Geometry check sheet. Reference: the model listing, model coordinates, mm. A direction names the side the tool comes from. Give positions to 0.01 mm unless a question says otherwise; leave off trailing zeros. Loops run counter-clockwise (first coordinate to the right, second up) from the corner with the lowest first, then second, coordinate; pieces in that order, holes last. Notation, with made-up numbers: (53, 19.5) -> (85, 19.5) arc R22 ccw to (85, 57.5) -> close; hole circle Ø9 at (41.25, -29). An arc over 180 degrees is marked (long way). Answer in a Markdown table with one row per item. Add a question column.
```python
from build123d import *

# Parameters (mm, degrees)
MAIN_BODY_DEPTH     = 7
SKETCH3_W           = 32
SKETCH3_H           = 20
BOSS_EXTRUDE2_DEPTH = 7
SKETCH4_W           = 28.5
SKETCH4_H           = 4
BOSS_EXTRUDE3_DEPTH = 6.5
SKETCH7_W           = 32
SKETCH7_H           = 7
BOSS_EXTRUDE4_DEPTH = 15
SKETCH10_R          = 1.9
CUT_EXTRUDE5_DEPTH  = 7
SKETCH13_W          = 10
SKETCH13_H          = 20
BOSS_EXTRUDE5_DEPTH = 10
SKETCH14_W          = 40
SKETCH14_H          = 20
SKETCH14_R          = 1.9
BOSS_EXTRUDE6_DEPTH = 6
SKETCH17_W          = 71
SKETCH17_H          = 5
BOSS_EXTRUDE7_DEPTH = 7
SKETCH19_R          = 1.25
CUT_EXTRUDE7_DEPTH  = 7
SKETCH21_R          = 1.6
CUT_EXTRUDE9_DEPTH  = 4
SKETCH22_R          = 1.9
CUT_EXTRUDE10_DEPTH = 7
SKETCH15_R          = 2.5621
DUE_MOUNT_DEPTH     = 172.689399789


with BuildPart() as part:
    # Sketch2 → Main body (new body)
    with BuildSketch(Plane(origin=(0, 0, 0), x_dir=(1, 0, 0), z_dir=(0, 1, 0))):
        with BuildLine():
            Line((0, 0), (71, 0))
            Line((71, 0), (71, -120))
            ThreePointArc((71, -120), (35.5, -155.5), (0, -120))
            Line((0, -120), (0, 0))
        make_face()
    extrude(amount=MAIN_BODY_DEPTH)

    # Sketch3 → Boss-Extrude2 (add)
    with BuildSketch(Plane(origin=(0, 7, 0), x_dir=(1, 0, 0), z_dir=(0, 1, 0))):
        with Locations((35.5, 10)):
            Rectangle(SKETCH3_W, SKETCH3_H)
    extrude(amount=-BOSS_EXTRUDE2_DEPTH)

    # Sketch4 → Boss-Extrude3 (add)
    with BuildSketch(Plane(origin=(0, 7, 0), x_dir=(1, 0, 0), z_dir=(0, 1, 0))):
        with Locations((35.5, 18)):
            Rectangle(SKETCH4_W, SKETCH4_H)
    extrude(amount=BOSS_EXTRUDE3_DEPTH)

    # Sketch7 → Boss-Extrude4 (add)
    with BuildSketch(Plane(origin=(0, 0, -20), x_dir=(-1, 0, 0), z_dir=(0, 0, -1))):
        with Locations((-35.5, 3.5)):
            Rectangle(SKETCH7_W, SKETCH7_H)
    extrude(amount=BOSS_EXTRUDE4_DEPTH)

    # Sketch10 → Cut-Extrude5 (cut)
    with BuildSketch(Plane(origin=(0, 7, 0), x_dir=(1, 0, 0), z_dir=(0, 1, 0))):
        with Locations(Location((4, -120, 0), (0, 0, 270))):
            Circle(SKETCH10_R)
        with Locations(Location((4, -110, 0), (0, 0, 270))):
            Circle(SKETCH10_R)
        with Locations(Location((4, -100, 0), (0, 0, 270))):
            Circle(SKETCH10_R)
        with Locations(Location((4, -90, 0), (0, 0, 270))):
            Circle(SKETCH10_R)
        with Locations(Location((4, -80, 0), (0, 0, 270))):
            Circle(SKETCH10_R)
        with Locations(Location((4, -70, 0), (0, 0, 270))):
            Circle(SKETCH10_R)
        with Locations(Location((4, -60, 0), (0, 0, 270))):
            Circle(SKETCH10_R)
        with Locations(Location((4, -50, 0), (0, 0, 270))):
            Circle(SKETCH10_R)
        with Locations(Location((4, -40, 0), (0, 0, 270))):
            Circle(SKETCH10_R)
        with Locations(Location((4, -30, 0), (0, 0, 270))):
            Circle(SKETCH10_R)
        with Locations(Location((4, -20, 0), (0, 0, 270))):
            Circle(SKETCH10_R)
        with Locations(Location((4, -10, 0), (0, 0, 270))):
            Circle(SKETCH10_R)
        with Locations(Location((8.220199781, -135.75, 0), (0, 0, 270))):
            Circle(SKETCH10_R)
        with Locations(Location((19.75, -147.279800219, 0), (0, 0, 270))):
            Circle(SKETCH10_R)
        with Locations(Location((35.5, -151.5, 0), (0, 0, 270))):
            Circle(SKETCH10_R)
        with Locations(Location((51.25, -147.279800219, 0), (0, 0, 270))):
            Circle(SKETCH10_R)
        with Locations(Location((62.779800219, -135.75, 0), (0, 0, 270))):
            Circle(SKETCH10_R)
        with Locations(Location((67, -120, 0), (0, 0, 270))):
            Circle(SKETCH10_R)
        with Locations(Location((67, -10, 0), (0, 0, 270))):
            Circle(SKETCH10_R)
        with Locations(Location((67, -20, 0), (0, 0, 270))):
            Circle(SKETCH10_R)
        with Locations(Location((67, -30, 0), (0, 0, 270))):
            Circle(SKETCH10_R)
        with Locations(Location((67, -40, 0), (0, 0, 270))):
            Circle(SKETCH10_R)
        with Locations(Location((67, -50, 0), (0, 0, 270))):
            Circle(SKETCH10_R)
        with Locations(Location((67, -60, 0), (0, 0, 270))):
            Circle(SKETCH10_R)
        with Locations(Location((67, -70, 0), (0, 0, 270))):
            Circle(SKETCH10_R)
        with Locations(Location((67, -80, 0), (0, 0, 270))):
            Circle(SKETCH10_R)
        with Locations(Location((67, -90, 0), (0, 0, 270))):
            Circle(SKETCH10_R)
        with Locations(Location((67, -100, 0), (0, 0, 270))):
            Circle(SKETCH10_R)
        with Locations(Location((67, -110, 0), (0, 0, 270))):
            Circle(SKETCH10_R)
    extrude(amount=-CUT_EXTRUDE5_DEPTH, mode=Mode.SUBTRACT)

    # Sketch13 → Boss-Extrude5 (add)
    with BuildSketch(Plane.XZ):
        with Locations((35.5, 120)):
            Rectangle(SKETCH13_W, SKETCH13_H)
        with Locations((35.5, 5)):
            Rectangle(SKETCH13_W, SKETCH13_H)
    extrude(amount=BOSS_EXTRUDE5_DEPTH)

    # Sketch14 → Boss-Extrude6 (add)
    # profile 1 of 2: a face of its own
    with BuildSketch(Plane.XZ.offset(10)):
        with Locations((35.5, 120)):
            Rectangle(SKETCH14_W, SKETCH14_H)
        with Locations(Location((23, 125, 0), (0, 0, 270))):
            Circle(SKETCH14_R, mode=Mode.SUBTRACT)
        with Locations(Location((23, 115, 0), (0, 0, 90))):
            Circle(SKETCH14_R, mode=Mode.SUBTRACT)
        with Locations(Location((48, 125, 0), (0, 0, 90))):
            Circle(SKETCH14_R, mode=Mode.SUBTRACT)
        with Locations(Location((48, 115, 0), (0, 0, 270))):
            Circle(SKETCH14_R, mode=Mode.SUBTRACT)
    # profile 2 of 2: a face of its own
    with BuildSketch(Plane.XZ.offset(10)):
        with Locations((35.5, 5)):
            Rectangle(SKETCH14_W, SKETCH14_H)
        with Locations(Location((48, 0, 0), (0, 0, 270))):
            Circle(SKETCH14_R, mode=Mode.SUBTRACT)
        with Locations(Location((48, 10, 0), (0, 0, 90))):
            Circle(SKETCH14_R, mode=Mode.SUBTRACT)
        with Locations(Location((23, 0, 0), (0, 0, 90))):
            Circle(SKETCH14_R, mode=Mode.SUBTRACT)
        with Locations(Location((23, 10, 0), (0, 0, 270))):
            Circle(SKETCH14_R, mode=Mode.SUBTRACT)
    extrude(amount=BOSS_EXTRUDE6_DEPTH)

    # Sketch17 → Boss-Extrude7 (add)
    with BuildSketch(Plane(origin=(0, 7, 0), x_dir=(1, 0, 0), z_dir=(0, 1, 0))):
        with Locations((35.5, 2.5)):
            Rectangle(SKETCH17_W, SKETCH17_H)
    extrude(amount=-BOSS_EXTRUDE7_DEPTH)

    # Sketch19 → Cut-Extrude7 (cut)
    with BuildSketch(Plane(origin=(0, 7, 0), x_dir=(1, 0, 0), z_dir=(0, 1, 0))):
        with Locations(Location((11.25, -8, 0), (0, 0, 270))):
            Circle(SKETCH19_R)
        with Locations(Location((59.75, -8, 0), (0, 0, 270))):
            Circle(SKETCH19_R)
    extrude(amount=-CUT_EXTRUDE7_DEPTH, mode=Mode.SUBTRACT)

    # Sketch21 → Cut-Extrude9 (cut)
    with BuildSketch(Plane(origin=(0, 0, -20), x_dir=(-1, 0, 0), z_dir=(0, 0, -1))):
        with Locations((-45.915, 10)):
            Circle(SKETCH21_R)
        with Locations((-25.085, 10)):
            Circle(SKETCH21_R)
    extrude(amount=-CUT_EXTRUDE9_DEPTH, mode=Mode.SUBTRACT)

    # Sketch22 → Cut-Extrude10 (cut)
    with BuildSketch(Plane(origin=(0, 7, 0), x_dir=(1, 0, 0), z_dir=(0, 1, 0))):
        with Locations(Location((23.5, 28, 0), (0, 0, 270))):
            Circle(SKETCH22_R)
        with Locations(Location((47.5, 28, 0), (0, 0, 270))):
            Circle(SKETCH22_R)
    extrude(amount=-CUT_EXTRUDE10_DEPTH, mode=Mode.SUBTRACT)

    # Sketch15 → DUE mount (cut, through all)
    with BuildSketch(Plane.XZ):
        with Locations(Location((24.3162, 46.805, 0), (0, 0, 270))):
            Circle(SKETCH15_R)
        with Locations(Location((52.2562, 46.805, 0), (0, 0, 270))):
            Circle(SKETCH15_R)
        with Locations(Location((57.3362, 97.605, 0), (0, 0, 270))):
            Circle(SKETCH15_R)
        with Locations(Location((9.0762, 97.605, 0), (0, 0, 270))):
            Circle(SKETCH15_R)
    extrude(amount=-DUE_MOUNT_DEPTH, mode=Mode.SUBTRACT)


solid = part.part
```
1. Release check for a two-part mould opening along X. For faces 1 (the face through (45.814, 3.549, -27.123)), 2 (the face through (15.5, -13, 5)), 3 (the face through (49.156, -12.958, 123.492)), 4 (the face through (35, -16, 5)) record: released by +X, released by -X, zero draft, split by the parting line, or undercut.
2. Sectioned sample at D-D (z = -28). Enter the section's corners in (x, y), plus the area to 3 significant figures.
3. Gauge pin test, flat ends, axial feed: pin 1 Ø6 at (x, z) = (54.5, 119.5) entering from +Y; pin 2 Ø3.5 at (x, z) = (67, 110) entering from +Y; pin 3 Ø2 at (x, z) = (49, 47.5) entering from -Y; pin 4 Ø1.8 at (y, z) = (-13.5, 1) entering from -X. Record the tip position at first contact, or that the pin passes through.
4. Sectioned sample at A-A (z = 20). Enter the section's corners in (x, y), plus the area to 3 significant figures.
5. Sectioned sample at B-B (y = -13.75). Count the separate pieces of the cut face and the enclosed holes in it, plus the area to 3 significant figures.
6. Access from +Z, -Z, +X, -X, +Y, -Y to the whole of each face (thin tool, end or side, straight path). Record for faces 5 (the face through (49.855, -12.958, 9.588)), 6 (the face through (35, -10, 110)), 7 (the face through (15.5, -13, 120)), 8 (the face through (48, -10, 120)), 9 (the face through (4.571, 3.549, 51.812)).
7. Sectioned sample at C-C (z = 151.5). Enter the section's corners in (x, y), plus the area to 3 significant figures.
8. Material ranges on L1, parallel to X at y = 5.25, z = 70; L2, parallel to Y at x = 25, z = 4; L3, parallel to Y at x = 45.5, z = -24, recorded low to high. Write a range as from..to.
Response:
| question | item | result |
|---|---|---|
| 1 | face 1 | undercut |
| 1 | face 2 | released by -X |
| 1 | face 3 | undercut |
| 1 | face 4 | zero draft |
| 2 | outline | (19.5, 0) -> (21.6, 0) -> (21.6, 7) -> (19.5, 7) -> close; (25.4, 0) -> (45.6, 0) -> (45.6, 7) -> (25.4, 7) -> close; (49.4, 0) -> (51.5, 0) -> (51.5, 7) -> (49.4, 7) -> close |
| 2 | area | 171 mm2 |
| 3 | pin 1 | stops at y = 7 |
| 3 | pin 2 | passes through |
| 3 | pin 3 | stops at y = 0 |
| 3 | pin 4 | stops at x = 15.5 |
| 4 | outline | (0, 0) -> (2.1, 0) -> (2.1, 7) -> (0, 7) -> close; (5.9, 0) -> (65.1, 0) -> (65.1, 7) -> (5.9, 7) -> close; (68.9, 0) -> (71, 0) -> (71, 7) -> (68.9, 7) -> close |
| 4 | area | 444 mm2 |
| 5 | separate pieces | 2 |
| 5 | enclosed holes | 8 |
| 5 | area | 1,510 mm2 |
| 6 | face 5 | -Y |
| 6 | face 6 | +X, -X, -Y |
| 6 | face 7 | +Z, -Z, -X, -Y |
| 6 | face 8 | +Z, -Z, +X |
| 6 | face 9 | +Y, -Y |
| 7 | outline | (19.13, 0) -> (33.6, 0) -> (33.6, 7) -> (19.13, 7) -> close; (37.4, 0) -> (51.87, 0) -> (51.87, 7) -> (37.4, 7) -> close |
| 7 | area | 203 mm2 |
| 8 | L1 | x = 0..2.1, 5.9..65.1, 68.9..71 |
| 8 | L2 | y = -16..-10, 0..7 |
| 8 | L3 | y = 0..7 |
